Design review of the part built by this model. Coordinates are the model's own, in mm. A direction names the side the tool comes from. Round coordinates to 2 decimals unless told otherwise and drop trailing zeros. Order: outer loops, then holes, each group sorted by start corner. A loop starts at its lowest first (then second) coordinate and runs counter-clockwise, first axis right, second up. Notation, with made-up numbers: (39, -14.75) - (98, -14.75) arc R20 ccw to (98, 2.25) - close; hole circle Ø8 at (29, 21). An arc over 180 degrees is marked (long way). Write item = value, one per line.
from build123d import *

# Parameters (mm, degrees)
SKETCH1_R                = 6.335999901
BOSS_EXTRUDE1_DEPTH      = 1.524
CUT_EXTRUDE1_DEPTH       = 10.089134474
FILLET1_R                = 0.191999997
CIRPATTERN1_COUNT        = 15
FILLET1_OF_CIRPATTERN1_R = 0.191999997
CUT_EXTRUDE2_DEPTH       = 10.455482489
CUT_EXTRUDE2_DEPTH_BACK  = 10.455482489
SKETCH4_R                = 3.55
SKETCH6_W                = 1.4
SKETCH6_H                = 0.7
CUT_EXTRUDE3_DEPTH       = 10.455482489


with BuildPart() as part:
    # Sketch1 → Boss-Extrude1 (new, symmetric)
    with BuildSketch(Plane.XY):
        with Locations(Location((0, 0, 0), (0, 0, 180))):
            Circle(SKETCH1_R)
    extrude(amount=BOSS_EXTRUDE1_DEPTH, both=True)

    # Sketch3 → Cut-Extrude1 (cut, symmetric)
    with BuildSketch(Plane.XY):
        with BuildLine():
            Line((-0.428414679, 4.780843037), (0.428414679, 4.780843037))
            ThreePointArc((0.428414679, 4.780843037), (1.010780942, 6.170659573), (2.288190337, 6.970012879))
            ThreePointArc((2.288190337, 6.970012879), (0, 7.335999901), (-2.288190337, 6.970012879))
            ThreePointArc((-2.288190337, 6.970012879), (-1.010780942, 6.170659573), (-0.428414679, 4.780843037))
        make_face()
    cut_extrude1 = extrude(amount=CUT_EXTRUDE1_DEPTH, both=True, mode=Mode.SUBTRACT)

    # Fillet1
    fillet1_edges = [part.edges().sort_by_distance(p)[0] for p in [
        (-0.428414679, 4.780843037, 0),
        (0.428414679, 4.780843037, 0),
    ]]
    fillet(fillet1_edges, radius=FILLET1_R)

    # CirPattern1: Cut-Extrude1 ×15 about axis
    cirpattern1_axis = Axis((0, 0, 0), (0, 0, 1))
    for i in range(1, CIRPATTERN1_COUNT):
        add(cut_extrude1.rotate(cirpattern1_axis, i * 360 / CIRPATTERN1_COUNT), mode=Mode.SUBTRACT)

    # Fillet1 of CirPattern1
    fillet1_of_cirpattern1_edges = [part.edges().sort_by_distance(p)[0] for p in [
        (-2.335920332, 4.193265492, 0),
        (-1.553167764, 4.541769388, 0),
        (-3.839524138, 2.880634248, 0),
        (-3.26619339, 3.517382552, 0),
        (-4.67923934, 1.069915174, 0),
        (-4.414464507, 1.884808318, 0),
        (-4.70987155, -0.925801954, 0),
        (-4.799434606, -0.073666397, 0),
        (-3.926124182, -2.761439514, 0),
        (-4.354538861, -2.019403523, 0),
        (-2.463514275, -4.119599094, 0),
        (-3.156703787, -3.615967434, 0),
        (-0.574940369, -4.765442566, 0),
        (-1.41304595, -4.587297726, 0),
        (1.41304595, -4.587297726, 0),
        (0.574940369, -4.765442566, 0),
        (3.156703787, -3.615967434, 0),
        (2.463514275, -4.119599094, 0),
        (4.354538861, -2.019403523, 0),
        (3.926124182, -2.761439514, 0),
        (4.799434606, -0.073666397, 0),
        (4.70987155, -0.925801954, 0),
        (4.414464507, 1.884808318, 0),
        (4.67923934, 1.069915174, 0),
        (3.26619339, 3.517382552, 0),
        (3.839524138, 2.880634248, 0),
        (1.553167764, 4.541769388, 0),
        (2.335920332, 4.193265492, 0),
    ]]
    fillet(fillet1_of_cirpattern1_edges, radius=FILLET1_OF_CIRPATTERN1_R)

    # Sketch4 → Cut-Extrude2 (cut, two sides: drawn at the far end of the back side and taken through both)
    with BuildSketch(Plane.XY.offset(1.524).offset(-CUT_EXTRUDE2_DEPTH_BACK)):
        Circle(SKETCH4_R)
    extrude(amount=CUT_EXTRUDE2_DEPTH + CUT_EXTRUDE2_DEPTH_BACK, mode=Mode.SUBTRACT)

    # Sketch6 → Cut-Extrude3 (cut, through all)
    with BuildSketch(Plane.XY.offset(1.524)):
        with Locations((0, 3.830301711)):
            Rectangle(SKETCH6_W, SKETCH6_H)
        with Locations((0, -3.830301711)):
            Rectangle(SKETCH6_W, SKETCH6_H)
    extrude(amount=-CUT_EXTRUDE3_DEPTH, mode=Mode.SUBTRACT)


solid = part.part
Item 1: For faces 1 (the face through (-5.67, 0.07, 0.02)), 2 (the face through (3.863, -4.177, 0.021)), 3 (the face through (-5.207, -2.243, 0.021)), list the 3-axis set-ups (+Z, -Z, +X, -X, +Y, -Y) from which the entire face can be reached by the end or side of a thin tool; tool diameter is ignored.
Data:
face_1 = +Z, -Z, -X
face_2 = +Z, -Z, -Y
face_3 = +Z, -Z
Item 2: Take a section at B-B, the plane y = -0.5. State the section outline as (x, z) points.
Data:
outline = (-4.75, -1.52) - (-3.51, -1.52) - (-3.51, 1.52) - (-4.75, 1.52) - close; (3.51, -1.52) - (4.75, -1.52) - (4.75, 1.52) - (3.51, 1.52) - close
Item 3: For line 1 along Y through (x, z) = (-5.5, -0.25); line 2 along Y through (x, z) = (4.25, 1.3); line 3 along X through (y, z) = (4, -0.2), list the stretches that pass through material, from the lowest coordinate up. Write a range as [from, to].
Data:
line_1 = [-2.25, -1.23], [0.02, 1.12], [2.78, 3.15]
line_2 = [-4.34, -3.03], [-2.2, 3.13]
line_3 = [-3.62, -0.7], [0.7, 3.62]
Item 4: Insertion check: P1, Ø0.6, axis at y = -3.5, z = -0.5, coming from the +X side; P2, Ø0.8, axis at y = -3.5, z = 0.5, coming from the -X side; P3, Ø1, axis at x = 4, z = 0.5, coming from the -Y side. Each pin has a flat end and moves straight along its axis. Give the tip position at first contact, or say it passes through.
Data:
P1 = 4.77
P2 = -4.82
P3 = -4.41
Item 5: The part is to be moulded in two halves that separate along Y. For faces 4 (the face through (0, -4.18, 0)), 5 (the face through (1.83, -5.387, 0.021)), 6 (the face through (0.66, 5.63, 0.02)), say which applies: +Y half, -Y half, draft (parallel to the pull), parting line (faces both ways), or undercut.
Data:
face_4 = undercut
face_5 = -Y half
face_6 = +Y half
Item 6: Take a section at A-A, the plane y = 2.25. State the section outline as (x, z) points.
Data:
outline = (-5.02, -1.52) - (-2.75, -1.52) - (-2.75, 1.52) - (-5.02, 1.52) - close; (2.75, -1.52) - (5.02, -1.52) - (5.02, 1.52) - (2.75, 1.52) - close
